from build123d import *

# Parameters (mm, degrees)
SKETCH1_R           = 15
BOSS_EXTRUDE1_DEPTH = 50
SKETCH2_R           = 5
BOSS_EXTRUDE2_DEPTH = 20
SKETCH3_W           = 20
SKETCH3_H           = 48.158533428
CUT_EXTRUDE1_DEPTH  = 30
SKETCH4_W           = 29.182617016
SKETCH4_H           = 12.047974763
CUT_EXTRUDE4_DEPTH  = 30
SKETCH7_W           = 65.578145757
SKETCH7_H           = 22.973592685
CUT_EXTRUDE5_DEPTH  = 30
FILLET6_R           = 3.5
SKETCH9_R           = 4
CUT_EXTRUDE6_DEPTH  = 58.879184669
SKETCH11_R          = 4
CUT_EXTRUDE7_DEPTH  = 58.879184669


with BuildPart() as part:
    # Sketch1 → Boss-Extrude1 (new body)
    with BuildSketch(Plane(origin=(0, 0, 0), x_dir=(1, 0, 0), z_dir=(0, 1, 0))):
        with Locations(Location((0, 0, 0), (0, 0, 90))):
            Circle(SKETCH1_R)
    extrude(amount=BOSS_EXTRUDE1_DEPTH)

    # Sketch2 → Boss-Extrude2 (add)
    with BuildSketch(Plane.XZ):
        with Locations(Location((0, 0, 0), (0, 0, 270))):
            Circle(SKETCH2_R)
    extrude(amount=BOSS_EXTRUDE2_DEPTH)

    # Sketch3 → Cut-Extrude1 (cut)
    with BuildSketch(Plane(origin=(0, 50, 0), x_dir=(1, 0, 0), z_dir=(0, 1, 0))):
        Rectangle(SKETCH3_W, SKETCH3_H)
    extrude(amount=-CUT_EXTRUDE1_DEPTH, mode=Mode.SUBTRACT)

    # Sketch4 → Cut-Extrude4 (cut)
    with BuildSketch(Plane(origin=(0, 50, 0), x_dir=(1, 0, 0), z_dir=(0, 1, 0))):
        with Locations((0.622640913, 13.072097126)):
            Rectangle(SKETCH4_W, SKETCH4_H)
    cut_extrude4 = extrude(amount=-CUT_EXTRUDE4_DEPTH, mode=Mode.SUBTRACT)

    # Sketch7 → Cut-Extrude5 (cut)
    with BuildSketch(Plane(origin=(0, 50, 0), x_dir=(1, 0, 0), z_dir=(0, 1, 0))):
        with Locations((5.132045661, 17.636797086)):
            Rectangle(SKETCH7_W, SKETCH7_H)
    extrude(amount=-CUT_EXTRUDE5_DEPTH, mode=Mode.SUBTRACT)

    # Mirror1: Cut-Extrude4 across plane
    add(cut_extrude4.mirror(Plane.XY), mode=Mode.SUBTRACT)

    # Fillet6
    fillet6_edges = [part.edges().sort_by_distance(p)[0] for p in [
        (-11.84064125, 20, -6.150000743),
        (11.84064125, 20, -6.150000743),
        (-11.84064125, 50, -6.150000743),
        (11.84064125, 50, -6.150000743),
        (-11.620501285, 50, 7.048109744),
        (11.620501285, 50, 7.048109744),
        (-11.620501285, 20, 7.048109744),
        (11.620501285, 20, 7.048109744),
    ]]
    fillet(fillet6_edges, radius=FILLET6_R)

    # Sketch9 → Cut-Extrude6 (cut, through all)
    with BuildSketch(Plane(origin=(-10, 0, 0), x_dir=(0, 0, -1), z_dir=(1, 0, 0))):
        with Locations((0, 40)):
            Circle(SKETCH9_R)
    extrude(amount=-CUT_EXTRUDE6_DEPTH, mode=Mode.SUBTRACT)

    # Sketch11 → Cut-Extrude7 (cut, through all)
    with BuildSketch(Plane.ZY.offset(-10)):
        with Locations((0.4490545, 40)):
            Circle(SKETCH11_R)
    extrude(amount=-CUT_EXTRUDE7_DEPTH, mode=Mode.SUBTRACT)


solid = part.part
For this review, take the finished solid that the model builds, in its own axes (mm). A direction names the side the tool comes from. Give positions to 0.01 mm unless a question says otherwise; leave off trailing zeros. Write each loop counter-clockwise with the first axis right and the second up, starting at its lowest first coordinate (ties: lowest second). Pieces come first, ordered by that corner, then holes. Notation, with made-up numbers: (37.25, 16) -> (56.25, 16) arc R19 ccw to (56.25, 42) -> close; hole circle Ø11 at (79, -17). An arc over 180 degrees is marked (long way). Use CSV: the item, a comma, the result in double quotes.
Q1. For P1, Ø10, axis at y = -13, z = -3, coming from the +X side; P2, Ø5, axis at x = -7, z = 11, coming from the +Y side; P3, Ø2.5, axis at x = 11.5, y = 33, coming from the +Z side, all flat-tipped, find the tip position at first contact; note any pin that passes through.
Conclusion:
P1,"x = 5"
P2,"y = 20"
P3,"z = 7.05"
Q2. Tool access review of faces 1 (the face through (10, 35, 1)), 2 (the face through (12, 35, -6.15)), 3 (the face through (-12, 35, 7.048)): name each direction out of +Z, -Z, +X, -X, +Y, -Y from which nothing blocks a thin tool from reaching the whole face with its end or side.
Conclusion:
face 1,"+Z, -Z, +Y"
face 2,"-Z, +X, -X, +Y"
face 3,"+Z, +X, -X, +Y"
Q3. Take a section at C-C, the plane x = 0. Write out the cut boundary in (y, z).
Conclusion:
outline,"(-20, -5) -> (0, -5) -> (0, -15) -> (20, -15) -> (20, 15) -> (0, 15) -> (0, 5) -> (-20, 5) -> close"
Q4. Take a section at A-A, the plane y = 25.5. Write out the cut boundary in (x, z), then the cut area to 3 significant figures.
Conclusion:
outline,"(-13.68, -6.15) -> (-10, -6.15) -> (-10, 7.05) -> (-13.24, 7.05) arc R15 ccw to start; (10, -6.15) -> (13.68, -6.15) arc R15 ccw to (13.24, 7.05) -> (10, 7.05) -> close"
area,"119 mm2"
Q5. Take a section at D-D, the plane y = 40. Write out the cut boundary in (x, z), then the cut area to 3 significant figures.
Conclusion:
outline,"(-14.46, -4) arc R15 ccw to (-13.68, -6.15) -> (-10, -6.15) -> (-10, -4) -> close; (-14.46, 4) -> (-10, 4) -> (-10, 7.05) -> (-13.24, 7.05) arc R15 ccw to start; (10, -6.15) -> (13.68, -6.15) arc R15 ccw to (14.57, -3.55) -> (10, -3.55) -> close; (10, 4.45) -> (14.33, 4.45) arc R15 ccw to (13.24, 7.05) -> (10, 7.05) -> close"
area,"41.5 mm2"
Q6. Take a section at B-B, the plane z = -1. Write out the cut boundary in (x, y).
Conclusion:
outline,"(-14.97, 0) -> (-4.9, 0) -> (-4.9, -20) -> (4.9, -20) -> (4.9, 0) -> (14.97, 0) -> (14.97, 36.27) -> (10, 36.27) -> (10, 20) -> (-10, 20) -> (-10, 36.13) -> (-14.97, 36.13) -> close; (-14.97, 43.87) -> (-10, 43.87) -> (-10, 50) -> (-14.97, 50) -> close; (10, 43.73) -> (14.97, 43.73) -> (14.97, 50) -> (10, 50) -> close"
Q7. Mouldability with a two-part tool opening along Z and no side actions: class faces 4 (the face through (-0.66, 13.539, 14.985)), 5 (the face through (-4, 0, 4)), 6 (the face through (12.467, 40.176, -3.547)), 7 (the face through (-12, 49, 6)) as pulls with the +Z half, pulls with the -Z half, needs draft (parallel to the pull), parting line crosses it, or undercut.
Conclusion:
face 4,"parting line crosses it"
face 5,"needs draft"
face 6,"undercut"
face 7,"pulls with the +Z half"
Q8. To check wall thickness, follow probe 1 along Y at (x, z) = (-11.45, 0); probe 2 along Y at (x, z) = (-4.5, -4.5); probe 3 along Z at (x, y) = (-12.7, 40). State the ranges of each line that lie inside material, in increasing order. Write a range as [from, to].
Conclusion:
probe 1,"[0, 36], [44, 50]"
probe 2,"[0, 20]"
probe 3,"[-6.15, -4], [4, 7.05]"
